```python
from build123d import *

# Parameters (mm, degrees)
F1_DEPTH  = 2
F2_W      = 22
F2_H      = 28
F3_DEPTH  = 1
F4_W      = 15
F4_H      = 21.1
F5_DEPTH  = 2.5
F6_W      = 5.5
F6_H      = 2
F7_DEPTH  = 5
F8_W      = 3
F8_H      = 3
F9_DEPTH  = 1
F10_R     = 1.5
F11_DEPTH = 2.5
F12_W     = 8
F12_H     = 1
F13_DEPTH = 15
F15_DEPTH = 49
F16_SIZE  = 2
F17_R     = 2
F18_W     = 8.038238
F18_H     = 1
F19_DEPTH = 0.5


with BuildPart() as f1:
    # F0 (on Top) → F1 (new body)
    with BuildSketch(Plane.XY):
        Polygon((-15, 61), (-15, 0), (15, 0), (15, 61), (3, 61), (3, 81), (-3, 81), (-3, 61), align=None)
    extrude(amount=F1_DEPTH)

    # F2 (on face) → F3 (join)
    with BuildSketch(Plane.XY.offset(2)):
        with Locations((0, 25)):
            Rectangle(F2_W, F2_H)
    extrude(amount=F3_DEPTH)

    # F4 (on face) → F5 (join)
    with BuildSketch(Plane.XY.offset(3)):
        with Locations((0, 26.65)):
            Rectangle(F4_W, F4_H)
    extrude(amount=F5_DEPTH)

    # F6 (on face) → F7 (join)
    with BuildSketch(Plane.XY.offset(2)):
        with Locations((3.25, 41)):
            Rectangle(F6_W, F6_H)
    extrude(amount=F7_DEPTH)

    # F8 (on face) → F9 (join)
    with BuildSketch(Plane.XY.offset(2)):
        with Locations((-0.5, 76.4)):
            Rectangle(F8_W, F8_H)
    extrude(amount=F9_DEPTH)

    # F10 (on face) → F11 (join)
    with BuildSketch(Plane.XY.offset(2)):
        with Locations((3.5, 7.5)):
            Circle(F10_R)
    extrude(amount=F11_DEPTH)

    # F12 (on face) → F13 (join)
    with BuildSketch(Plane(origin=(0, 0, 0), x_dir=(1, 0, 0), z_dir=(0, 0, -1))):
        with Locations((8.55, -4.5)):
            Rectangle(F12_W, F12_H)
        with Locations((-8.55, -4.5)):
            Rectangle(F12_W, F12_H)
        with Locations((8.55, -57)):
            Rectangle(F12_W, F12_H)
        with Locations((-8.55, -57)):
            Rectangle(F12_W, F12_H)
    extrude(amount=F13_DEPTH)

    # F14 (on face) → F15 (join)
    with BuildSketch(Plane.XZ.offset(-56.5)):
        with BuildLine():
            Line((15.53212, -9.6), (15.53212, -8.6))
            ThreePointArc((15.53212, -8.6), (8.55, -2.1), (1.56788, -8.6))
            Line((1.56788, -8.6), (1.56788, -9.6))
            ThreePointArc((1.56788, -9.6), (8.55, -16.1), (15.53212, -9.6))
        make_face()
        with BuildLine():
            ThreePointArc((-15.53212, -9.6), (-8.55, -16.1), (-1.56788, -9.6))
            Line((-1.56788, -9.6), (-1.56788, -8.6))
            ThreePointArc((-1.56788, -8.6), (-8.55, -2.1), (-15.53212, -8.6))
            Line((-15.53212, -8.6), (-15.53212, -9.6))
        make_face()
    extrude(amount=F15_DEPTH)

    # F16
    f16_edges = [f1.edges().sort_by_distance(p)[0] for p in [
        (-3, 61, 1),
        (3, 61, 1),
        (3, 81, 1),
        (-3, 81, 1),
    ]]
    chamfer(f16_edges, length=F16_SIZE)

    # F17
    f17_edges = [f1.edges().sort_by_distance(p)[0] for p in [
        (15, 61, 1),
        (-15, 61, 1),
        (15, 0, 1),
        (-15, 0, 1),
    ]]
    fillet(f17_edges, radius=F17_R)

    # F18 (on face) → F19 (join)
    with BuildSketch(Plane(origin=(-15.53212, 0, 0), x_dir=(0, -1, 0), z_dir=(-1, 0, 0))):
        with Locations((-32.501247, -9.1)):
            Rectangle(F18_W, F18_H)
    extrude(amount=F19_DEPTH)


solid = f1.part
```
Work out the finished part from the listing and answer in its coordinate system (mm). A direction names the side the tool comes from. Coordinates: 2 decimals unless noted, no trailing zeros. Write each loop counter-clockwise with the first axis right and the second up, starting at its lowest first coordinate (ties: lowest second). Pieces come first, ordered by that corner, then holes. Notation, with made-up numbers: (-25, 25.25) - (17, 25.25) arc R8 cw to (17, 40.25) - close; hole circle Ø7 at (23.5, 44). An arc over 180 degrees is marked (long way). Answer as a JSON object with one key per item and string values.
Q1. Find section B-B (z = 1). Write down the section's boundary in (x, y), plus the area to 3 significant figures.
Results list:
{"outline": "(-15, 2) arc R2 ccw to (-13, 0) - (13, 0) arc R2 ccw to (15, 2) - (15, 59) arc R2 ccw to (13, 61) - (5, 61) - (3, 63) - (3, 79) - (1, 81) - (-1, 81) - (-3, 79) - (-3, 63) - (-5, 61) - (-13, 61) arc R2 ccw to (-15, 59) - close", "area": "1,950 mm^2"}
Q2. For a pull along X with two mould halves and no side action, classify faces 1 (the flat face through (-7.5, 27, 4)), 2 (the cylindrical face through (8.4, 32.3, -16.1)), 3 (the cylindrical face through (8.7, 32.3, -2.1)), 4 (the flat face through (3, 40, 4)) as pulls with the +X half, pulls with the -X half, needs draft (parallel to the pull), parting line crosses it, or undercut.
Results list:
{"face 1": "pulls with the -X half", "face 2": "undercut", "face 3": "undercut", "face 4": "needs draft"}
Q3. Consider L1, parallel to Y at x = 6, z = -12.75; L2, parallel to Z at x = 1, y = 20.5; L3, parallel to Y at x = 14, z = -6.75. Determine where each line is inside the solid, lowest interval first. Write a range as from..to.
Results list:
{"L1": "y = 4..5, 7.5..57.5", "L2": "z = 0..5.5", "L3": "y = 7.5..56.5"}
Q4. Find section D-D (y = 71). Write down the section's boundary in (x, z).
Results list:
{"outline": "(-3, 0) - (3, 0) - (3, 2) - (-3, 2) - close"}
Q5. Which of the six approach directions +Z, -Z, +X, -X, +Y, -Y give full straight-line access (tool end or side, diameter ignored) to faces 5 (the flat face through (7.5, 27, 4)), 6 (the flat face through (0.5, 41, 4)), 7 (the flat face through (3, 71, 1))?
Results list:
{"face 5": "+Z, +X, +Y, -Y", "face 6": "+Z, -X", "face 7": "+Z, -Z, +X, +Y"}
Q6. Find section C-C (x = 14). Write down the section's boundary in (y, z).
Results list:
{"outline": "(0.27, 0) - (60.73, 0) - (60.73, 2) - (0.27, 2) - close; (7.5, -13.49) - (56.5, -13.49) - (56.5, -4.71) - (7.5, -4.71) - close"}
Q7. Find section A-A (y = 14). Write down the section's boundary in (x, z).
Results list:
{"outline": "(-15.53, -9.6) arc R7 ccw to (-1.57, -9.6) - (-1.57, -8.6) arc R7 ccw to (-15.53, -8.6) - close; (-15, 0) - (15, 0) - (15, 2) - (11, 2) - (11, 3) - (-11, 3) - (-11, 2) - (-15, 2) - close; (1.57, -9.6) arc R7 ccw to (15.53, -9.6) - (15.53, -8.6) arc R7 ccw to (1.57, -8.6) - close"}
Q8. Given pin 1 Ø1.6 at (y, z) = (71.5, 1) entering from +X; pin 2 Ø3.5 at (x, z) = (-13.5, -6.5) entering from +Y; pin 3 Ø6 at (x, z) = (-7.5, -1) entering from +Y; pin 4 Ø1 at (y, z) = (59.5, -7) entering from +X, each flat-ended and moving along its own axis, determine where each tip first touches the part or whether it passes through.
Results list:
{"pin 1": "stops at x = 3", "pin 2": "stops at y = 57.5", "pin 3": "stops at y = 61.33", "pin 4": "passes through"}
